```python
from build123d import *

# Parameters (mm, degrees)
SKETCH1_R          = 4.2
SKETCH1_R_2        = 3.2
BASE_FLANGE1_DEPTH = 10


# Sheet-metal steps are written as plain solids
with BuildPart() as part:
    # Sketch1 → Base-Flange1 (new body)
    with BuildSketch(Plane(origin=(0, 0, 0), x_dir=(1, 0, 0), z_dir=(0, 1, 0))):
        with BuildLine():
            Line((-132.5, 122.5), (132.5, 122.5))
            ThreePointArc((132.5, 122.5), (139.571067812, 119.571067812), (142.5, 112.5))
            Line((142.5, 112.5), (142.5, -112.5))
            ThreePointArc((142.5, -112.5), (139.571067812, -119.571067812), (132.5, -122.5))
            Line((132.5, -122.5), (-132.5, -122.5))
            ThreePointArc((-132.5, -122.5), (-139.571067812, -119.571067812), (-142.5, -112.5))
            Line((-142.5, -112.5), (-142.5, 112.5))
            ThreePointArc((-142.5, 112.5), (-139.571067812, 119.571067812), (-132.5, 122.5))
        make_face()
        with Locations(Location((120, 40, 0), (0, 0, 270))):
            Circle(SKETCH1_R, mode=Mode.SUBTRACT)
        with Locations(Location((120, -40, 0), (0, 0, 270))):
            Circle(SKETCH1_R, mode=Mode.SUBTRACT)
        with Locations(Location((-120, 40, 0), (0, 0, 270))):
            Circle(SKETCH1_R, mode=Mode.SUBTRACT)
        with Locations(Location((-120, -40, 0), (0, 0, 270))):
            Circle(SKETCH1_R, mode=Mode.SUBTRACT)
        with Locations(Location((-120, 100, 0), (0, 0, 270))):
            Circle(SKETCH1_R, mode=Mode.SUBTRACT)
        with Locations(Location((-50, 100, 0), (0, 0, 270))):
            Circle(SKETCH1_R, mode=Mode.SUBTRACT)
        with Locations(Location((50, 100, 0), (0, 0, 270))):
            Circle(SKETCH1_R, mode=Mode.SUBTRACT)
        with Locations(Location((120, 100, 0), (0, 0, 270))):
            Circle(SKETCH1_R, mode=Mode.SUBTRACT)
        with Locations(Location((120, -100, 0), (0, 0, 270))):
            Circle(SKETCH1_R, mode=Mode.SUBTRACT)
        with Locations(Location((50, -100, 0), (0, 0, 270))):
            Circle(SKETCH1_R, mode=Mode.SUBTRACT)
        with Locations(Location((-50, -100, 0), (0, 0, 270))):
            Circle(SKETCH1_R, mode=Mode.SUBTRACT)
        with Locations(Location((-120, -100, 0), (0, 0, 270))):
            Circle(SKETCH1_R, mode=Mode.SUBTRACT)
        with Locations(Location((31, 0, 0), (0, 0, 270))):
            Circle(SKETCH1_R_2, mode=Mode.SUBTRACT)
        with Locations(Location((15.5, -26.846787517, 0), (0, 0, 270))):
            Circle(SKETCH1_R_2, mode=Mode.SUBTRACT)
        with Locations(Location((-15.5, -26.846787517, 0), (0, 0, 270))):
            Circle(SKETCH1_R_2, mode=Mode.SUBTRACT)
        with Locations(Location((-31, 0, 0), (0, 0, 270))):
            Circle(SKETCH1_R_2, mode=Mode.SUBTRACT)
        with Locations(Location((-15.5, 26.846787517, 0), (0, 0, 270))):
            Circle(SKETCH1_R_2, mode=Mode.SUBTRACT)
        with Locations(Location((15.5, 26.846787517, 0), (0, 0, 270))):
            Circle(SKETCH1_R_2, mode=Mode.SUBTRACT)
    extrude(amount=-BASE_FLANGE1_DEPTH)


solid = part.part
```
Here's how the part is built. I have some questions about the finished solid (model axes, mm). Give positions to 0.01 mm unless a question says otherwise; leave off trailing zeros. Write each loop counter-clockwise with the first axis right and the second up, starting at its lowest first coordinate (ties: lowest second). Pieces come first, ordered by that corner, then holes. Notation, with made-up numbers: M 21,17.5 L 53,17.5 A15 ccw 53,28.5 Z; hole C -31.5,73.5 d4. An arc over 180 degrees is marked long. Put each result on its own line as item: value. Start each with the question number.
Item 1: If we section it at D-D, the plane x = 31: Write out the boundary of the cut face in (y, z).
Item 2: If we section it at B-B, the plane x = -15.5: Write out the boundary of the cut face in (y, z), then the cut area to 3 significant figures.
Item 3: If we section it at A-A, the plane z = -100: Write out the boundary of the cut face in (x, y).
Item 4: Thinking about a two-plate mould opening in Z: for faces 1 (the flat face through (2, 0, -2)), 2 (the cylindrical face through (-123.726, -4.93, -38.062)), 3 (the cylindrical face through (-139.65, -4.93, -119.49)), which applies, +Z half, -Z half, draft (parallel to the pull), parting line (faces both ways), or undercut?
Item 5: If we section it at C-C, the plane z = 40: Write out the boundary of the cut face in (x, y).
Item 6: I need wall thicknesses on L1, parallel to X at y = -3, z = 100; L2, parallel to X at y = -7.75, z = -40; L3, parallel to X at y = -5, z = 0. Which ranges of each line are inside material? Lowest first, please. Write a range as from..to.
Item 7: Will this pin go through, and if not, where does the flat tip stop? pin 1 (6.5 mm diameter, centred on x = 120, z = -100, fed in from +Y).
Values:
1. outline: M -10,-122.5 L 0,-122.5 L 0,-3.2 L -10,-3.2 Z; M -10,3.2 L 0,3.2 L 0,122.5 L -10,122.5 Z
2. outline: M -10,-122.5 L 0,-122.5 L 0,-30.05 L -10,-30.05 Z; M -10,-23.65 L 0,-23.65 L 0,23.65 L -10,23.65 Z; M -10,30.05 L 0,30.05 L 0,122.5 L -10,122.5 Z
2. area: 2,320 mm²
3. outline: M -142.5,-10 L -124.2,-10 L -124.2,0 L -142.5,0 Z; M -115.8,-10 L -54.2,-10 L -54.2,0 L -115.8,0 Z; M -45.8,-10 L 45.8,-10 L 45.8,0 L -45.8,0 Z; M 54.2,-10 L 115.8,-10 L 115.8,0 L 54.2,0 Z; M 124.2,-10 L 142.5,-10 L 142.5,0 L 124.2,0 Z
4. face 1: draft
4. face 2: undercut
4. face 3: -Z half
5. outline: M -142.5,-10 L -124.2,-10 L -124.2,0 L -142.5,0 Z; M -115.8,-10 L 115.8,-10 L 115.8,0 L -115.8,0 Z; M 124.2,-10 L 142.5,-10 L 142.5,0 L 124.2,0 Z
6. L1: -142.5..-124.2, -115.8..-54.2, -45.8..45.8, 54.2..115.8, 124.2..142.5
6. L2: -142.5..-124.2, -115.8..115.8, 124.2..142.5
6. L3: -142.5..-34.2, -27.8..27.8, 34.2..142.5
7. pin 1: through
